The drawing under review shows one solid part. Ordinate dimensions are in mm from its lowest x, y, z. Round coordinates to 2 decimals unless told otherwise and drop trailing zeros. Write each loop counter-clockwise with the first axis right and the second up, starting at its lowest first coordinate (ties: lowest second). Pieces come first, ordered by that corner, then holes. Notation, with made-up numbers: (-32.75, 9) -> (15.25, 9) arc R14 cw to (15.25, 25) -> close; hole circle Ø9 at (74, -33). An arc over 180 degrees is marked (long way). Write item = value, one per line. Start each with the question number.
Item 1: For pin 1 Ø1.9 at (x, z) = (9.5, 33) entering from +Y; pin 2 Ø3 at (x, z) = (14.5, 10.5) entering from -Y; pin 3 Ø11 at (x, z) = (25, 22) entering from +Y; pin 4 Ø1.2 at (x, y) = (45, 2.5) entering from +Z, all flat-tipped, find the tip position at first contact; note any pin that passes through.
Item 2: Add section B-B, the plane z = 27.5. State the section outline as (x, y) points, then the cut area to 4 significant figures.
Item 3: Add section D-D, the plane x = 36. State the section outline as (y, z) points.
Item 4: Add section A-A, the plane x = 9.5. State the section outline as (y, z) points, then the cut area to 3 significant figures.
Item 5: Add section C-C, the plane y = 2.35. State the section outline as (x, z) points, then the cut area to 3 significant figures.
Item 6: To check wall thickness, follow L1, parallel to X at y = 1.1, z = 33; L2, parallel to X at y = 1.4, z = 32; L3, parallel to X at y = 1.65, z = 12.5. State the ranges of each line that lie inside material, in increasing order.
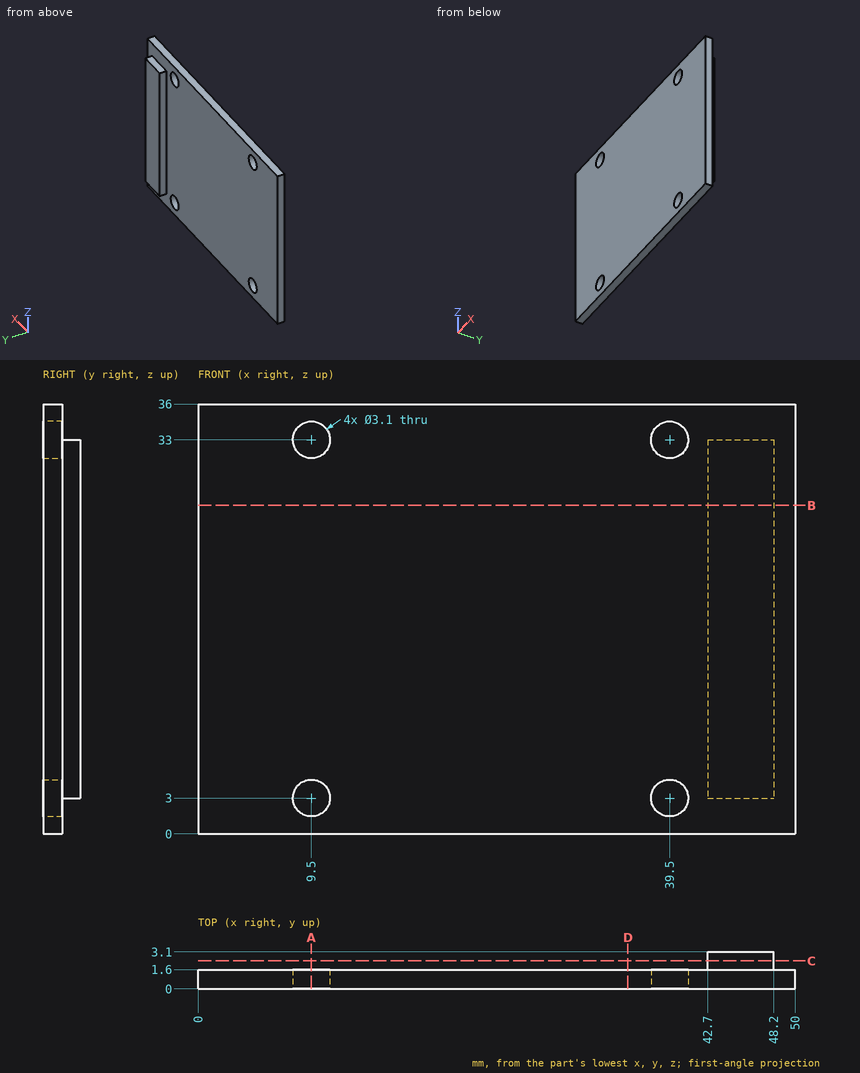
Result set:
q1.pin_1 = through
q1.pin_2 = 0
q1.pin_3 = 1.6
q1.pin_4 = 33
q2.outline = (0, 0) -> (50, 0) -> (50, 1.6) -> (48.2, 1.6) -> (48.2, 3.1) -> (42.7, 3.1) -> (42.7, 1.6) -> (0, 1.6) -> close
q2.area = 88.25 mm²
q3.outline = (0, 0) -> (1.6, 0) -> (1.6, 36) -> (0, 36) -> close
q4.outline = (0, 0) -> (1.6, 0) -> (1.6, 1.45) -> (0, 1.45) -> close; (0, 4.55) -> (1.6, 4.55) -> (1.6, 31.45) -> (0, 31.45) -> close; (0, 34.55) -> (1.6, 34.55) -> (1.6, 36) -> (0, 36) -> close
q4.area = 47.7 mm²
q5.outline = (42.7, 3) -> (48.2, 3) -> (48.2, 33) -> (42.7, 33) -> close
q5.area = 165 mm²
q6.L1 = 0 to 7.95, 11.05 to 37.95, 41.05 to 50
q6.L2 = 0 to 8.32, 10.68 to 38.32, 40.68 to 50
q6.L3 = 42.7 to 48.2
